Geometry check sheet. Reference: the model listing, model coordinates, mm. A direction names the side the tool comes from. Give positions to 0.01 mm unless a question says otherwise; leave off trailing zeros. Write each loop counter-clockwise with the first axis right and the second up, starting at its lowest first coordinate (ties: lowest second). Pieces come first, ordered by that corner, then holes. Notation, with made-up numbers: (14.5, 51.5) - (67.5, 51.5) arc R16 ccw to (67.5, 74.5) - close; hole circle Ø3 at (-20.75, -33.75). An arc over 180 degrees is marked (long way). One line per question, with ' | ' between items. Start each with the question number.
Q1. Set-up check for faces 1 (the face through (38.1, 46, -16)), 2 (the face through (16, 54, -25.4)), 3 (the face through (19, 13, -6.35)): record each of +Z, -Z, +X, -X, +Y, -Y from which the full face is reachable in a straight line by a thin tool's end or side.
Q2. Section check A-A on y = 63.5. Record the boundary of the cut face in (x, z) (3 decimals).
Q3. Section check D-D on x = 5.5. Record the boundary of the cut face in (y, z), and give its area (3 significant figures).
Q4. Release check for a two-part mould opening along X. For faces 4 (the face through (33, 76.2, -16)), 5 (the face through (4.643, 66.177, -28.619)), 6 (the face through (2.86, 73.48, -3.22)) record: +X half, -X half, draft (parallel to the pull), parting line (faces both ways), or undercut.
Q5. Section check B-B on x = 25. Record the boundary of the cut face in (y, z), and give its area (3 significant figures).
Q6. Thickness scan on L1, parallel to Z at x = 15, y = 49.5; L2, parallel to X at y = 55, z = -22; L3, parallel to Y at x = 3.5, z = -12.5. Record the ranges inside material, lowest first. Write a range as [from, to].
Q7. Gauge pin test, flat ends, axial feed: P1, Ø5.5, axis at x = 6.35, y = 63.5, coming from the -Z side; P2, Ø4, axis at x = 23.5, z = -23, coming from the +Y side; P3, Ø1.5, axis at x = 20, z = -11.5, coming from the -Y side; P4, Ø20.5, axis at x = 12.5, y = 13, coming from the -Z side. Record the tip position at first contact, or that the pin passes through.
Q8. Section check C-C on z = -23. Record the boundary of the cut face in (x, y).
```python
from build123d import *

# Parameters (mm, degrees)
SKETCH1_W           = 38.1
SKETCH1_H           = 76.2
BOSS_EXTRUDE1_DEPTH = 31.75
SKETCH3_W           = 25.4
SKETCH3_H           = 76.2
CUT_EXTRUDE2_DEPTH  = 31.75
SKETCH4_W           = 25.4
SKETCH4_H           = 25.4
CUT_EXTRUDE3_DEPTH  = 89.44526556
SKETCH5_W           = 31.75
SKETCH5_H           = 6.35
BOSS_EXTRUDE2_DEPTH = 50.8
SKETCH6_R           = 3.175
CUT_EXTRUDE4_DEPTH  = 50.8
FILLET2_R           = 9.525
SKETCH7_W           = 31.75
SKETCH7_H           = 19.05
BOSS_EXTRUDE3_DEPTH = 6.35


with BuildPart() as part:
    # Sketch1 → Boss-Extrude1 (new body)
    with BuildSketch(Plane.XY):
        with Locations((19.05, 38.1)):
            Rectangle(SKETCH1_W, SKETCH1_H)
    extrude(amount=-BOSS_EXTRUDE1_DEPTH)

    # Sketch3 → Cut-Extrude2 (cut)
    with BuildSketch(Plane.ZY):
        with Locations((-19.05, 38.1)):
            Rectangle(SKETCH3_W, SKETCH3_H)
    extrude(amount=-CUT_EXTRUDE2_DEPTH, mode=Mode.SUBTRACT)

    # Sketch4 → Cut-Extrude3 (cut, through all)
    with BuildSketch(Plane.ZY.offset(-31.75)):
        with Locations((-19.05, 12.7)):
            Rectangle(SKETCH4_W, SKETCH4_H)
    extrude(amount=-CUT_EXTRUDE3_DEPTH, mode=Mode.SUBTRACT)

    # Sketch5 → Boss-Extrude2 (add)
    with BuildSketch(Plane(origin=(0, 76.2, 0), x_dir=(1, 0, 0), z_dir=(0, 1, 0))):
        with Locations((15.875, 28.575)):
            Rectangle(SKETCH5_W, SKETCH5_H)
    extrude(amount=-BOSS_EXTRUDE2_DEPTH)

    # Sketch6 → Cut-Extrude4 (cut)
    with BuildSketch(Plane(origin=(0, 0, -31.75), x_dir=(-1, 0, 0), z_dir=(0, 0, -1))):
        with Locations((-6.35, 63.5)):
            Circle(SKETCH6_R)
    extrude(amount=-CUT_EXTRUDE4_DEPTH, mode=Mode.SUBTRACT)

    # Fillet2
    fillet2_edges = [part.edges().sort_by_distance(p)[0] for p in [
        (0, 76.2, -3.175),
        (0, 76.2, -28.575),
    ]]
    fillet(fillet2_edges, radius=FILLET2_R)

    # Sketch7 → Boss-Extrude3 (add)
    with BuildSketch(Plane(origin=(0, 25.4, 0), x_dir=(-1, 0, 0), z_dir=(0, -1, 0))):
        with Locations((-15.875, 15.875)):
            Rectangle(SKETCH7_W, SKETCH7_H)
    extrude(amount=-BOSS_EXTRUDE3_DEPTH)


solid = part.part
```
Working result:
1) face 1: +Z, -Z, +X, +Y, -Y | face 2: -X, +Y | face 3: -Z, +X, -X, -Y
2) outline: (0, -31.75) - (3.175, -31.75) - (3.175, -25.4) - (0, -25.4) - close; (0, -6.35) - (3.175, -6.35) - (3.175, 0) - (0, 0) - close; (9.525, -31.75) - (38.1, -31.75) - (38.1, 0) - (9.525, 0) - (9.525, -6.35) - (31.75, -6.35) - (31.75, -25.4) - (9.525, -25.4) - close
3) outline: (0, -6.35) - (25.4, -6.35) - (25.4, -31.75) - (60.44, -31.75) - (60.44, -25.4) - (31.75, -25.4) - (31.75, -6.35) - (60.44, -6.35) - (60.44, 0) - (0, 0) - close; (66.56, -31.75) - (75.31, -31.75) - (75.31, -25.4) - (66.56, -25.4) - close; (66.56, -6.35) - (75.31, -6.35) - (75.31, 0) - (66.56, 0) - close | area: 838 mm2
4) face 4: draft | face 5: undercut | face 6: -X half
5) outline: (0, -6.35) - (25.4, -6.35) - (25.4, -31.75) - (76.2, -31.75) - (76.2, -25.4) - (31.75, -25.4) - (31.75, -6.35) - (76.2, -6.35) - (76.2, 0) - (0, 0) - close | area: 927 mm2
6) L1: z = [-31.75, -25.4], [-6.35, 0] | L2: x = [31.75, 38.1] | L3: y = [25.4, 31.75]
7) P1: passes through | P2: stops at y = 31.75 | P3: stops at y = 25.4 | P4: stops at z = -6.35
8) outline: (0, 25.4) - (38.1, 25.4) - (38.1, 76.2) - (31.75, 76.2) - (31.75, 31.75) - (0, 31.75) - close
